For this review, take the finished solid that the model builds, in its own axes (mm). Give positions to 0.01 mm unless a question says otherwise; leave off trailing zeros. Order: outer loops, then holes, each group sorted by start corner. A loop starts at its lowest first (then second) coordinate and runs counter-clockwise, first axis right, second up.
Item 1: For P1, Ø1, axis at x = 0.5, y = 0.5, coming from the +Z side, flat-tipped, find the tip position at first contact; note if it passes through.
Item 2: The part is to be moulded in two halves that separate along X. For faces 1 (the flat face through (2, 2, -1.25)), 2 (the flat face through (0, 2, -1)), 3 (the cylindrical face through (2.3, 2.46, 2.25)), 4 (the flat face through (4.5, 2, -1)), say which applies: released by +X, released by -X, zero draft, split by the parting line, or undercut.
Item 3: Consider section D-D (y = 3.75). Give the boundary of the cut face in (x, z).
Item 4: Consider section C-C (z = 1.75). Give the boundary of the cut face in (x, y).
Item 5: Consider section B-B (y = -5). Give the boundary of the cut face in (x, z).
Item 6: For probe 1 along Y at (x, z) = (3.95, -0.7); probe 2 along X at (y, z) = (-3.25, -0.8); probe 3 along Z at (x, y) = (0.9, -4.25), list the stretches that pass through material, from the lowest coordinate up.
Item 7: Consider section A-A (x = 2.25). Give the boundary of the cut face in (y, z).
```python
from build123d import *

# Parameters (mm, degrees)
BOSS_EXTRUDE1_DEPTH = 5
SKETCH2_R           = 0.25
BOSS_EXTRUDE2_DEPTH = 7.5


with BuildPart() as part:
    # Sketch1 → Boss-Extrude1 (new body)
    with BuildSketch(Plane(origin=(0, 0, 0), x_dir=(1, 0, 0), z_dir=(0, 1, 0))):
        with BuildLine():
            Line((0, 1.25), (4.5, 1.25))
            Line((4.5, 1.25), (4.5, 0))
            ThreePointArc((4.5, 0), (2.25, -2.25), (0, 0))
            Line((0, 0), (0, 1.25))
        make_face()
    extrude(amount=BOSS_EXTRUDE1_DEPTH)

    # Sketch2 → Boss-Extrude2 (add)
    with BuildSketch(Plane.XZ):
        with Locations((1, -0.75)):
            Circle(SKETCH2_R)
        with Locations((3.5, -0.75)):
            Circle(SKETCH2_R)
        with Locations((2.25, 1.75)):
            Circle(SKETCH2_R)
    extrude(amount=BOSS_EXTRUDE2_DEPTH)


solid = part.part
```
Resolved:
1. P1: stops at z = 1.87
2. face 1: zero draft
2. face 2: released by -X
2. face 3: split by the parting line
2. face 4: released by +X
3. outline: (0, -1.25) - (4.5, -1.25) - (4.5, 0) arc R2.25 ccw to (0, 0) - close
4. outline: (0.84, 0) - (2, 0) - (2, -7.5) - (2.5, -7.5) - (2.5, 0) - (3.66, 0) - (3.66, 5) - (0.84, 5) - close
5. outline: circle Ø0.5 at (1, -0.75); circle Ø0.5 at (2.25, 1.75); circle Ø0.5 at (3.5, -0.75)
6. probe 1: y = 0 to 5
6. probe 2: x = 0.76 to 1.24, 3.26 to 3.74
6. probe 3: z = -0.98 to -0.52
7. outline: (-7.5, 1.5) - (0, 1.5) - (0, -1.25) - (5, -1.25) - (5, 2.25) - (0, 2.25) - (0, 2) - (-7.5, 2) - close
